from build123d import *

# Parameters (mm, degrees)
ESQUISSE1_W        = 30
ESQUISSE1_H        = 120
ESQUISSE1_R        = 2
ESQUISSE1_W_2      = 5
ESQUISSE1_H_2      = 5
BOSS_EXTRU_1_DEPTH = 5
CONG_1_R           = 10


with BuildPart() as part:
    # Esquisse1 → Boss.-Extru.1 (new body)
    with BuildSketch(Plane.XY):
        with Locations((-15, -60)):
            Rectangle(ESQUISSE1_W, ESQUISSE1_H)
        with Locations((-15, -10)):
            Circle(ESQUISSE1_R, mode=Mode.SUBTRACT)
        with Locations((-15, -87.5)):
            Circle(ESQUISSE1_R, mode=Mode.SUBTRACT)
        with Locations((-15, -112.5)):
            Circle(ESQUISSE1_R, mode=Mode.SUBTRACT)
        with Locations((-22.5, -10)):
            Rectangle(ESQUISSE1_W_2, ESQUISSE1_H_2, mode=Mode.SUBTRACT)
        with Locations((-7.5, -112.5)):
            Rectangle(ESQUISSE1_W_2, ESQUISSE1_H_2, mode=Mode.SUBTRACT)
        with Locations((-22.5, -112.5)):
            Rectangle(ESQUISSE1_W_2, ESQUISSE1_H_2, mode=Mode.SUBTRACT)
        with Locations((-22.5, -87.5)):
            Rectangle(ESQUISSE1_W_2, ESQUISSE1_H_2, mode=Mode.SUBTRACT)
        with Locations((-7.5, -87.5)):
            Rectangle(ESQUISSE1_W_2, ESQUISSE1_H_2, mode=Mode.SUBTRACT)
        with Locations((-7.5, -10)):
            Rectangle(ESQUISSE1_W_2, ESQUISSE1_H_2, mode=Mode.SUBTRACT)
    extrude(amount=BOSS_EXTRU_1_DEPTH)

    # Congé1
    cong_1_edges = [part.edges().sort_by_distance(p)[0] for p in [
        (-30, 0, 2.5),
        (0, 0, 2.5),
        (0, -120, 2.5),
        (-30, -120, 2.5),
    ]]
    fillet(cong_1_edges, radius=CONG_1_R)


solid = part.part
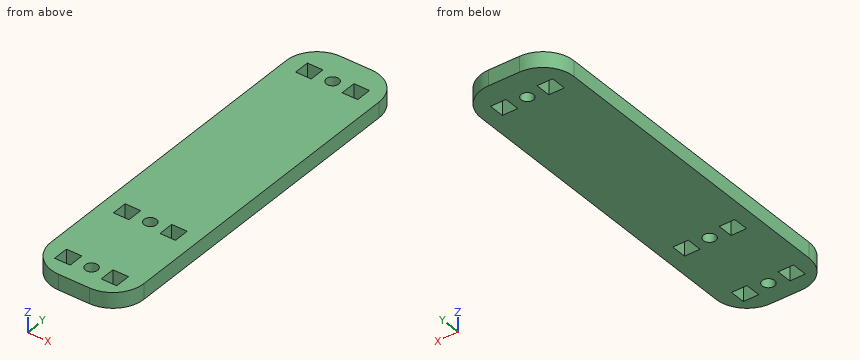
Can you work these out from the model? Positions are in its coordinate system, mm. Give positions to 0.01 mm unless a question says otherwise; leave off trailing zeros. Loops run counter-clockwise (first coordinate to the right, second up) from the corner with the lowest first, then second, coordinate; pieces in that order, holes last. Notation, with made-up numbers: (46.25, -38.75) -> (98.25, -38.75) arc R16 ccw to (98.25, -12.75) -> close; hole circle Ø5 at (10.25, 79.25). An arc over 180 degrees is marked (long way). Write item = value, one per line.
1) Will these pins go through, and if not, where does the flat tip stop? pin 1 (2.5 mm diameter, centred on y = -112, z = 2.5, fed in from +X); pin 2 (2.5 mm diameter, centred on x = -23, z = 1.5, fed in from -Y).
Check result:
pin_1 = -0.03
pin_2 = -119.85
2) Suppose I cut it at D-D on x = -27. Write out the boundary of the cut face in (y, z), then the cut area to 3 significant figures.
Check result:
outline = (-117.14, 0) -> (-2.86, 0) -> (-2.86, 5) -> (-117.14, 5) -> close
area = 571 mm2
3) Suppose I cut it at A-A on x = -15. Write out the boundary of the cut face in (y, z), then the cut area to 3 significant figures.
Check result:
outline = (-120, 0) -> (-114.5, 0) -> (-114.5, 5) -> (-120, 5) -> close; (-110.5, 0) -> (-89.5, 0) -> (-89.5, 5) -> (-110.5, 5) -> close; (-85.5, 0) -> (-12, 0) -> (-12, 5) -> (-85.5, 5) -> close; (-8, 0) -> (0, 0) -> (0, 5) -> (-8, 5) -> close
area = 540 mm2
4) I need wall thicknesses on L1, parallel to Y at x = -15, z = 1.95; L2, parallel to Y at x = -20.5, z = 0.3; L3, parallel to Y at x = -28.25, z = 1.6. Which ranges of each line are inside material? Lowest first, please. Write a range as from..to.
Check result:
L1 = -120..-114.5, -110.5..-89.5, -85.5..-12, -8..0
L2 = -119.99..-115, -110..-90, -85..-12.5, -7.5..-0.01
L3 = -115.65..-4.35
5) Suppose I cut it at B-B on z = 0.95. Give the number of separate pieces and of enclosed holes in the cut face, then the cut area to 3 significant figures.
Check result:
separate_pieces = 1
enclosed_holes = 9
area = 3,330 mm2
6) Suppose I cut it at C-C on x = -22.5. Write out the boundary of the cut face in (y, z), then the cut area to 3 significant figures.
Check result:
outline = (-119.68, 0) -> (-115, 0) -> (-115, 5) -> (-119.68, 5) -> close; (-110, 0) -> (-90, 0) -> (-90, 5) -> (-110, 5) -> close; (-85, 0) -> (-12.5, 0) -> (-12.5, 5) -> (-85, 5) -> close; (-7.5, 0) -> (-0.32, 0) -> (-0.32, 5) -> (-7.5, 5) -> close
area = 522 mm2
